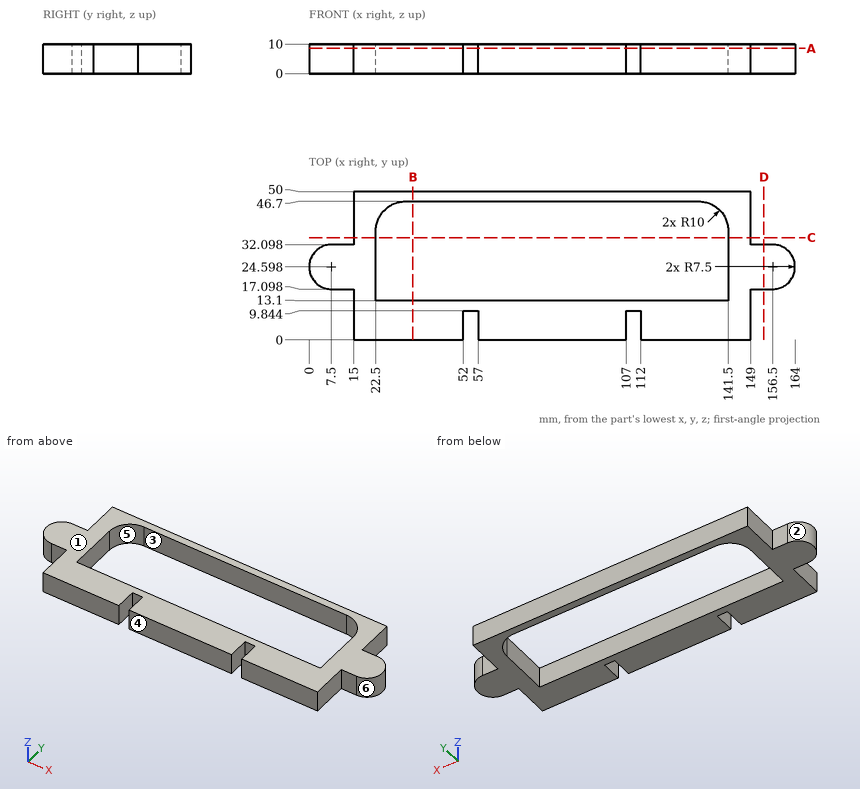
Geometry check sheet. Reference: drawing and pictorial views, mm from the part's lowest x, y, z. A direction names the side the tool comes from. Coordinates: 2 decimals unless noted, no trailing zeros. Order: outer loops, then holes, each group sorted by start corner. A loop starts at its lowest first (then second) coordinate and runs counter-clockwise, first axis right, second up.
Item 1: Access from +Z, -Z, +X, -X, +Y, -Y to the whole of each face (thin tool, end or side, straight path). Record for the marked faces 5 and 6.
Filled in:
face 5: +Z, -Z
face 6: +Z, -Z, +X
Item 2: Depth check by flat-ended pin: pin 1 (3 mm diameter, centred on x = 50.5, y = 12.5, fed in from -Z); pin 2 (4 mm diameter, centred on x = 152, z = 7, fed in from +Y); pin 3 (1.5 mm diameter, centred on y = 20.5, z = 4, fed in from +X); pin 4 (2 mm diameter, centred on y = 16, z = 5.5, fed in from -X). Enter the tip coordinate at first touch or a pass-through.
Filled in:
pin 1: stops at z = 0
pin 2: stops at y = 32.1
pin 3: stops at x = 163.21
pin 4: stops at x = 15
Item 3: Section check C-C, the plane y = 34.5. Enter the section's corners in (x, z).
Filled in:
outline: (15, 0) - (22.5, 0) - (22.5, 10) - (15, 10) - close; (141.5, 0) - (149, 0) - (149, 10) - (141.5, 10) - close
Item 4: Section check D-D, the plane x = 153.5. Enter the section's corners in (y, z), then the cut area to 3 significant figures.
Filled in:
outline: (17.1, 0) - (32.1, 0) - (32.1, 10) - (17.1, 10) - close
area: 150 mm2
Item 5: Section check A-A, the plane z = 8.5. Enter the section's corners in (x, y) (1 decimal), then the cut area to 3 significant figures.
Filled in:
outline: (7.5, 17.1) - (15, 17.1) - (15, 0) - (52, 0) - (52, 9.8) - (57, 9.8) - (57, 0) - (107, 0) - (107, 9.8) - (112, 9.8) - (112, 0) - (149, 0) - (149, 17.1) - (156.5, 17.1) arc R7.5 ccw to (156.5, 32.1) - (149, 32.1) - (149, 50) - (15, 50) - (15, 32.1) - (7.5, 32.1) arc R7.5 ccw to start; hole (22.5, 13.1) - (141.5, 13.1) - (141.5, 36.7) arc R10 ccw to (131.5, 46.7) - (32.5, 46.7) arc R10 ccw to (22.5, 36.7) - close
area: 3,050 mm2
Item 6: Release check for a two-part mould opening along Y. For the marked faces 1, 2, 3 and 4 record: +Y half, -Y half, draft (parallel to the pull), parting line (faces both ways), or undercut.
Filled in:
face 1: draft
face 2: parting line
face 3: undercut
face 4: -Y half
Item 7: Material ranges on L1, parallel to X at y = 7, z = 6; L2, parallel to X at y = 37.5, z = 5.25; L3, parallel to Y at x = 122, z = 7.75, recorded low to high.
Filled in:
L1: x = 15 to 52, 57 to 107, 112 to 149
L2: x = 15 to 22.53, 141.47 to 149
L3: y = 0 to 13.1, 46.7 to 50
Item 8: Section check B-B, the plane x = 35. Enter the section's corners in (y, z), then the cut area to 3 significant figures.
Filled in:
outline: (0, 0) - (13.1, 0) - (13.1, 10) - (0, 10) - close; (46.7, 0) - (50, 0) - (50, 10) - (46.7, 10) - close
area: 164 mm2
